Part print with two shaded views. Sizes in mm from the minimum x, y, z corner. A direction names the side the tool comes from. Give positions to 0.01 mm unless a question says otherwise; leave off trailing zeros. Write each loop counter-clockwise with the first axis right and the second up, starting at its lowest first coordinate (ties: lowest second). Pieces come first, ordered by that corner, then holes. Notation, with made-up numbers: (-26.5, 50.5) -> (-6.5, 50.5) arc R11 cw to (-6.5, 56.5) -> close; hole circle Ø1 at (50.5, 35). An arc over 180 degrees is marked (long way). Answer in a Markdown table with one row per item. Add a question column.
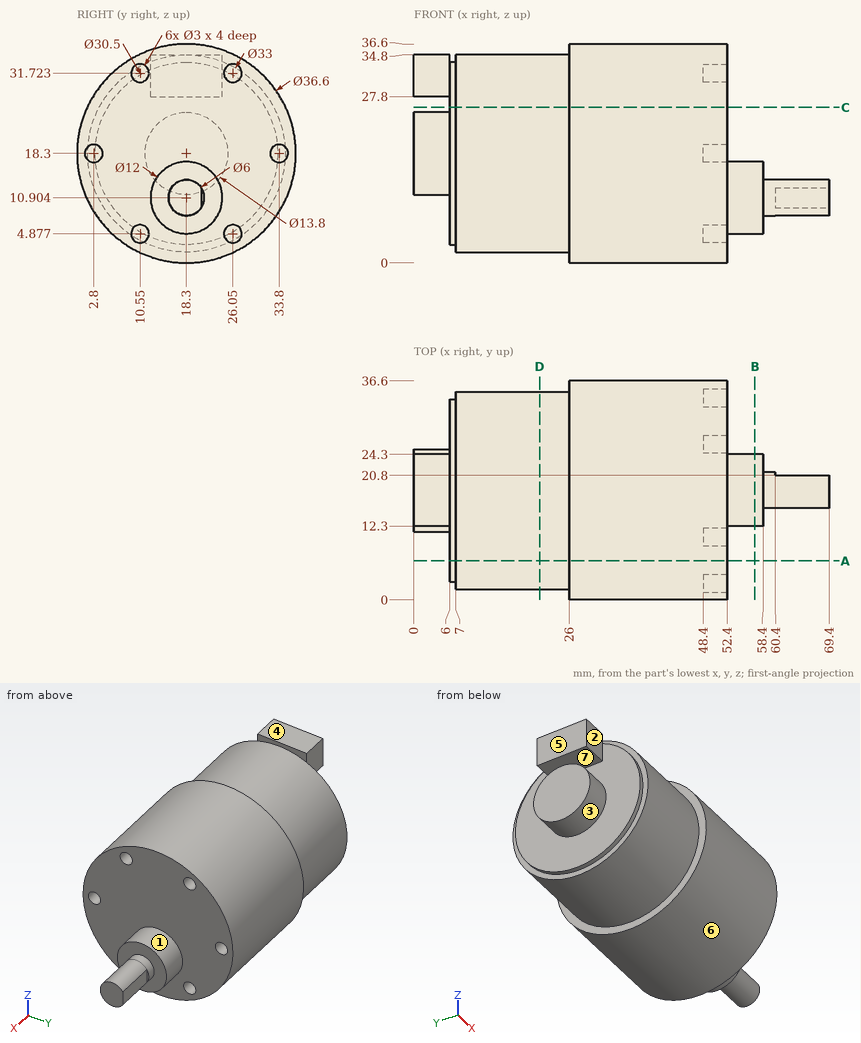
Item 1: Slice it at A-A, the plane y = 6.5. List the corners of the cut face in (x, z).
Item 2: Slice it at B-B, the plane x = 57. List the corners of the cut face in (y, z), then the cut area to 3 significant figures.
Item 3: Mould opens along Z. For the marked faces 5, 6 and 7 say: released by +Z, released by -Z, zero draft, split by the parting line, or undercut.
Item 4: Which spindle directions (+Z, -Z, +X, -X, +Y, -Y) get a long thin tool onto all of the face, cutting with end or side? Do the marked faces 1, 2, 3 and 4. Say none if no direction does.
Item 5: Slice it at D-D, the plane x = 21. List the corners of the cut face in (y, z).
Item 6: Slice it at C-C, the plane z = 26. List the corners of the cut face in (x, y).
Item 7: Drop flat-ended pins along their axis: pin 1 Ø2 at (x, y) = (22, 26) entering from -Z; pin 2 Ø3 at (x, y) = (8, 28) entering from +Z; pin 3 Ø10 at (x, z) = (11.5, 29.5) entering from +Y. Give the stop position or say it passes through.
Item 8: Probe L1, parallel to Z at x = 51, y = 26 (1 decimal); L2, parallel to X at y = 9, z = 31.5; L3, parallel to X at y = 27, z = 31.5. List the from-to ranges inside material, lowest first. Write a range as from..to.
Answer key:
| question | item | result |
|---|---|---|
| 1 | outline | (6, 8.64) -> (7, 8.64) -> (7, 6.77) -> (26, 6.77) -> (26, 4.31) -> (52.4, 4.31) -> (52.4, 32.29) -> (26, 32.29) -> (26, 29.83) -> (7, 29.83) -> (7, 27.96) -> (6, 27.96) -> close |
| 2 | outline | circle Ø12 at (18.3, 10.9) |
| 2 | area | 113 mm² |
| 3 | face 5 | zero draft |
| 3 | face 6 | split by the parting line |
| 3 | face 7 | undercut |
| 4 | face 1 | +X |
| 4 | face 2 | +Z, -X, -Y |
| 4 | face 3 | -X |
| 4 | face 4 | +Z, -X, +Y, -Y |
| 5 | outline | circle Ø33 at (18.3, 18.3) |
| 6 | outline | (6, 5.14) -> (7, 5.14) -> (7, 3.71) -> (26, 3.71) -> (26, 1.7) -> (52.4, 1.7) -> (52.4, 34.9) -> (26, 34.9) -> (26, 32.89) -> (7, 32.89) -> (7, 31.46) -> (6, 31.46) -> close |
| 7 | pin 1 | stops at z = 3.22 |
| 7 | pin 2 | stops at z = 32.62 |
| 7 | pin 3 | stops at y = 33.59 |
| 8 | L1 | z = 1.7..3.4, 6.4..30.2, 33.2..34.9 |
| 8 | L2 | x = 7..52.4 |
| 8 | L3 | x = 7..48.4 |
